```python
from build123d import *

# Parameters (mm, degrees)
F1_W     = 4
F1_H     = 15
F1_W_2   = 6
F1_H_2   = 6
F1_H_3   = 45
F2_DEPTH = 36.25
F4_DEPTH = 12


# Not quite as in the source:
# - a feature names something its author has since deleted; it is built from what else it names


with BuildPart() as f2:
    # F1 (on Front) → F2 (new body)
    with BuildSketch(Plane.XZ):
        Polygon((24.125, -2), (24.125, 2), (-24.125, 2), (-24.125, -2), (-20.125, -2), (20.125, -2), align=None)
        with Locations((-22.125, -9.5)):
            Rectangle(F1_W, F1_H)
        with Locations((22.125, -9.5)):
            Rectangle(F1_W, F1_H)
        Polygon((24.125, -21), (24.125, -17), (20.125, -17), (6, -17), (6, -21), align=None)
        Polygon((6, -21), (6, -17), (-4, -17), (-4, -20.7), (-6, -20.7), (-6, -26.7), (-4, -26.7), (-4, -29.7), (-0.85, -29.7), (2, -29.7), (6, -29.7), align=None)
        Polygon((-20.125, -17), (-24.125, -17), (-30, -17), (-30, -29.7), (-26, -29.7), (-23.15, -29.7), (-20, -29.7), (-20, -26.7), (-18, -26.7), (-18, -20.7), (-20, -20.7), (-20, -17), align=None)
        Polygon((-4, -20.7), (-4, -17), (-12, -17), (-12, -20.7), (-6, -20.7), align=None)
        Polygon((-12, -17), (-20, -17), (-20, -20.7), (-18, -20.7), (-12, -20.7), align=None)
        with Locations((-15, -23.7)):
            Rectangle(F1_W_2, F1_H_2)
        with Locations((-9, -23.7)):
            Rectangle(F1_W_2, F1_H_2)
        Polygon((-12, -29.7), (-12, -26.7), (-18, -26.7), (-20, -26.7), (-20, -29.7), align=None)
        Polygon((-6, -26.7), (-12, -26.7), (-12, -29.7), (-4, -29.7), (-4, -26.7), align=None)
        Polygon((30, -17), (24.125, -17), (24.125, -21), (26, -21), (26, -74.7), (30, -74.7), align=None)
        with Locations((-28, -52.2)):
            Rectangle(F1_W, F1_H_3)
        with Locations((4, -52.2)):
            Rectangle(F1_W, F1_H_3)
    extrude(amount=-F2_DEPTH)

    # F1 (on Front) → F3 (revolve, cut)
    with BuildSketch(Plane.XZ):
        Polygon((-12, -17), (-20, -17), (-20, -20.7), (-18, -20.7), (-12, -20.7), align=None)
        with Locations((-15, -23.7)):
            Rectangle(F1_W_2, F1_H_2)
        Polygon((-12, -29.7), (-12, -26.7), (-18, -26.7), (-20, -26.7), (-20, -29.7), align=None)
    revolve(axis=Axis((-12, 0, -48.15), (0, 0, -1)), mode=Mode.SUBTRACT)

    # F1 (on Front) → F4 (join)
    with BuildSketch(Plane.XZ):
        Polygon((24.125, -2), (24.125, 2), (-24.125, 2), (-24.125, -2), (-20.125, -2), (20.125, -2), align=None)
        with Locations((22.125, -9.5)):
            Rectangle(F1_W, F1_H)
        with Locations((-22.125, -9.5)):
            Rectangle(F1_W, F1_H)
        Polygon((24.125, -21), (24.125, -17), (20.125, -17), (6, -17), (6, -21), align=None)
        Polygon((30, -17), (24.125, -17), (24.125, -21), (26, -21), (26, -74.7), (30, -74.7), align=None)
        with Locations((-28, -52.2)):
            Rectangle(F1_W, F1_H_3)
        with Locations((4, -52.2)):
            Rectangle(F1_W, F1_H_3)
    extrude(amount=F4_DEPTH)


solid = f2.part
```
Model file for the job. Use its own axes, mm. A direction names the side the tool comes from. Coordinates: 2 decimals unless noted, no trailing zeros. Order: outer loops, then holes, each group sorted by start corner. A loop starts at its lowest first (then second) coordinate and runs counter-clockwise, first axis right, second up. Notation, with made-up numbers: (-27.75, 3.5) -> (-17.75, 3.5) arc R22 cw to (-17.75, 32.5) -> close; hole circle Ø5 at (62.25, -36.5). An arc over 180 degrees is marked (long way). Answer as a JSON object with one key per item and string values. Group by question number.
1) Pull direction X, two halves, no side cores. Call faces 4 (the face through (-12, 8, -19)), 5 (the face through (0, 12, 2)), 6 (the face through (24.125, 12, -8)): +X half, -X half, draft (parallel to the pull), parting line (faces both ways), or undercut.
2) Drill centre lines: L1, parallel to X at y = 16.5, z = -64.5; L2, parallel to Z at x = -11, y = 19; L3, parallel to Z at x = 15, y = 0. Where is each one in solid material? Low to high.
3) Flat gauge pins, fed straight in: pin 1 (2 mm diameter, centred on x = -23, y = -8, fed in from -Z); pin 2 (9.5 mm diameter, centred on y = 24, z = -11, fed in from -X) (3 decimals); pin 3 (1.8 mm diameter, centred on x = -26, y = 9, fed in from +Z); pin 4 (8 mm diameter, centred on x = 9.5, z = -30, fed in from -Y). Where does each tip first touch, or does it go through?
4) Cut at B-B, the plane y = -1. Write the cut outline in (x, z) (3 decimals), then the cut area to 3 significant figures.
5) Which spindle directions (+Z, -Z, +X, -X, +Y, -Y) get a long thin tool onto all of the face, cutting with end or side? Do faces 1 (the face through (0, 0, -23)), 2 (the face through (-22, -6, -17)), 3 (the face through (-12, 8, -28)). Say none if no direction does.
6) Cut at A-A, the plane z = -24.5. Write the cut outline in (x, y).
7) Cut at D-D, the plane z = -40.5. Write the cut outline in (x, y), then the cut area to 3 significant figures.
8) Cut at C-C, the plane x = 16.5. Write the cut outline in (y, z), then the cut area to 3 significant figures.
Check values:
{
 "1": {"face 4": "undercut", "face 5": "draft", "face 6": "+X half"},
 "2": {"L1": "x = -30 to -26, 2 to 6, 26 to 30", "L2": "z = -29.7 to -17, -2 to 2", "L3": "z = -21 to -17, -2 to 2"},
 "3": {"pin 1": "stops at z = -17", "pin 2": "stops at x = -24.125", "pin 3": "stops at z = -17", "pin 4": "stops at y = -12"},
 "4": {"outline": "(-30, -74.7) -> (-26, -74.7) -> (-26, -29.7) -> (-30, -29.7) -> close; (-24.125, -17) -> (-20.125, -17) -> (-20.125, -2) -> (20.125, -2) -> (20.125, -17) -> (6, -17) -> (6, -21) -> (26, -21) -> (26, -74.7) -> (30, -74.7) -> (30, -17) -> (24.125, -17) -> (24.125, 2) -> (-24.125, 2) -> close; (2, -74.7) -> (6, -74.7) -> (6, -29.7) -> (2, -29.7) -> close", "area": "984 mm²"},
 "5": {"face 1": "-X, -Y", "face 2": "-Z, -X, -Y", "face 3": "-Z, -Y"},
 "6": {"outline": "(-30, 0) -> (-18, 0) arc R6 cw to (-6, 0) -> (6, 0) -> (6, 36.25) -> (-30, 36.25) -> close; (26, -12) -> (30, -12) -> (30, 36.25) -> (26, 36.25) -> close"},
 "7": {"outline": "(-30, -12) -> (-26, -12) -> (-26, 36.25) -> (-30, 36.25) -> close; (2, -12) -> (6, -12) -> (6, 36.25) -> (2, 36.25) -> close; (26, -12) -> (30, -12) -> (30, 36.25) -> (26, 36.25) -> close", "area": "579 mm²"},
 "8": {"outline": "(-12, -21) -> (36.25, -21) -> (36.25, -17) -> (-12, -17) -> close; (-12, -2) -> (36.25, -2) -> (36.25, 2) -> (-12, 2) -> close", "area": "386 mm²"}
}
